Geometry: final body of the model. Coordinates: model frame, mm. A direction names the side the tool comes from. Give positions to 0.01 mm unless a question says otherwise; leave off trailing zeros. Loops run counter-clockwise (first coordinate to the right, second up) from the corner with the lowest first, then second, coordinate; pieces in that order, holes last. Notation, with made-up numbers: (26, -7.75) -> (74, -7.75) arc R14 cw to (74, 5.25) -> close; hole circle Ø5 at (-14.5, 3.25). An arc over 180 degrees is marked (long way). One line per question, with ' | ' between items. Start each with the question number.
Item 1: Set-up query: faces 1 (the cylindrical face through (10.24, -21.994, -4.224)), 2 (the flat face through (14, 22.2, 0)), 3 (the flat face through (-20.32, 0, -5)). Return all of +Z, -Z, +X, -X, +Y, -Y with unobstructed straight access to the full face (end or side cutting, diameter ignored); none if empty.
Item 2: Section D-D on y = 0. Return loops of the section in (x, z), then the cut area to 3 significant figures.
Item 3: Section B-B on x = -12. Give the number of separate pieces and of enclosed holes in the cut face, then the cut area to 3 significant figures.
Item 4: Section A-A on z = 24. Return loops of the section in (x, y).
Item 5: Material intervals for line 1 along X through (y, z) = (20, -3); line 2 along Y through (x, z) = (0, 18); line 3 along Z through (x, y) = (16.5, -7.5), sorted ascending. Write a range as [from, to].
Item 6: Section C-C on x = 0. Return loops of the section in (y, z) (3 decimals), then the cut area to 3 significant figures.
Item 7: Pin query (flat end, axial travel): P1, Ø7, axis at x = 12.065, y = 20.32, coming from the +Z side; P2, Ø10, axis at x = 13, y = -20, coming from the +Z side; P3, Ø3, axis at x = 12.065, y = 20.32, coming from the +Z side; P4, Ø1, axis at x = 5, y = 31, coming from the -Z side. Return the tip coordinate at first contact, or that it passes through.
Item 8: Mould query, pull axis Y, two halves, no side actions, for faces 4 (the flat face through (-10, 22, 0)), 5 (the flat face through (-1, -27, -2.54)), 6 (the cylindrical face through (35.09, 34.86, 26.46)). Classes: released by +Y, released by -Y, zero draft, split by the parting line, or undercut.
Autodesk Fusion 360 part; units mm, degrees
sketch "Sketch1" plane through (0, 0, 0) normal (0, 0, 1) x (1, 0, 0)
  line L0 (39.37, 39.37) -> (-39.37, 39.37)
  line L1 (-39.37, 39.37) -> (-39.37, -39.37)
  line L2 (-39.37, -39.37) -> (39.37, -39.37)
  line L3 (39.37, -39.37) -> (39.37, 39.37)
  line L4 (39.37, 39.37) -> (-39.37, -39.37) construction
  line L5 (-39.37, 39.37) -> (39.37, -39.37) construction
  dimension "d9" = 78.74
  dimension "d10" = 78.74
extrude "Extrude1" add sketch "Sketch1" along normal blind 50.8
sketch "Sketch2" plane through (0, 0, 50.8) normal (0, 0, 1) x (-1, 0, 0)
  line L0 (-39.37, 39.37) -> (-39.37, -39.37)
  line L1 (-39.37, -39.37) -> (39.37, -39.37)
  line L2 (39.37, -39.37) -> (39.37, 39.37)
  line L3 (39.37, 39.37) -> (-39.37, 39.37)
  circle A0 centre (0, 0) radius 36.83
  dimension "d13" = 73.66
extrude "Extrude2" cut sketch "Sketch2" against normal up to surface (50.8 mm away) contours A0
sketch "Sketch3" plane through (0, 0, 0) normal (0, 0, -1) x (1, 0, 0)
  circle A0 centre (0, 0) radius 36.83
  line L0 (39.37, -39.37) -> (39.37, 39.37)
  line L1 (39.37, 39.37) -> (-39.37, 39.37)
  line L2 (-39.37, 39.37) -> (-39.37, -39.37)
  line L3 (-39.37, -39.37) -> (39.37, -39.37)
  line L4 (-39.37, 39.37) -> (39.37, 39.37)
  line L5 (39.37, 39.37) -> (39.37, -39.37)
  line L6 (39.37, -39.37) -> (-39.37, -39.37)
  line L7 (-39.37, -39.37) -> (-39.37, 39.37)
extrude "Extrude3" add sketch "Sketch3" along normal blind 2.54 contours A0 | L0 L1 L2 L3 L4 L5 L6 L7
sketch "Sketch4" plane through (0, 0, -2.54) normal (0, 0, -1) x (1, 0, 0)
  line L0 (-39.37, -39.37) -> (39.37, -39.37)
  line L1 (39.37, -39.37) -> (39.37, 39.37)
  line L2 (39.37, 39.37) -> (-39.37, 39.37)
  line L3 (-39.37, 39.37) -> (-39.37, -39.37)
  line L4 (-20.32, 26.035) -> (20.32, 26.035)
  line L5 (20.32, 26.035) -> (20.32, -26.035)
  line L6 (20.32, -26.035) -> (-20.32, -26.035)
  line L7 (-20.32, -26.035) -> (-20.32, 26.035)
  line L8 (-20.32, 26.035) -> (20.32, -26.035) construction
  line L9 (20.32, 26.035) -> (-20.32, -26.035) construction
  dimension "d18" = 40.64
  dimension "d19" = 52.07
extrude "Extrude4" add sketch "Sketch4" along normal blind 5.7912 contours L4 L5 L6 L7
sketch "Sketch5" plane through (0, 0, -8.3312) normal (0, 0, -1) x (1, 0, 0)
  line L0 (-20.32, -26.035) -> (20.32, -26.035)
  line L1 (20.32, -26.035) -> (20.32, 26.035)
  line L2 (20.32, 26.035) -> (-20.32, 26.035)
  line L3 (-20.32, 26.035) -> (-20.32, -26.035)
  line L4 (-12.065, 20.32) -> (12.065, 20.32)
  line L5 (12.065, 20.32) -> (12.065, -20.32)
  line L6 (12.065, -20.32) -> (-12.065, -20.32)
  line L7 (-12.065, -20.32) -> (-12.065, 20.32)
  line L8 (-12.065, 20.32) -> (12.065, -20.32) construction
  line L9 (12.065, 20.32) -> (-12.065, -20.32) construction
  circle A0 centre (12.065, -20.32) radius 2.4765
  circle A1 centre (-12.065, -20.32) radius 2.4765
  circle A2 centre (-12.065, 20.32) radius 2.4765
  circle A3 centre (12.065, 20.32) radius 2.4765
  dimension "d23" = 24.13
  dimension "d24" = 40.64
  dimension "d26" = 4.953
  dimension "d27" = 4.953
  dimension "d28" = 4.953
  dimension "d29" = 4.953
extrude "Extrude5" cut sketch "Sketch5" against normal up to surface (59.1312 mm away) contours L4 L7 A2 | L4 L7 A2 | L4 L5 A3 | L4 L5 A3 | L6 L7 A1 | L6 L7 A1 | L5 L6 A0 | L5 L6 A0
sketch "Sketch6" plane through (0, 0, 0) normal (0, 0, 1) x (-1, 0, 0)
  circle A0 centre (12.065, -20.32) radius 2.4765
  circle A1 centre (12.065, 20.32) radius 2.4765
  circle A2 centre (-12.065, -20.32) radius 2.4765
  circle A3 centre (-12.065, 20.32) radius 2.4765
  circle A4 centre (0, 0) radius 36.83
  line L0 (-12.065, 20.32) -> (12.065, 20.32)
  line L1 (12.065, 20.32) -> (12.065, -20.32)
  line L2 (12.065, -20.32) -> (-12.065, -20.32)
  line L3 (-12.065, -20.32) -> (-12.065, 20.32)
  circle A5 centre (-12.065, 20.32) radius 4.445
  circle A6 centre (12.065, 20.32) radius 4.445
  circle A7 centre (-12.065, -20.32) radius 4.445
  circle A8 centre (12.065, -20.32) radius 4.445
  dimension "d33" = 8.89
  dimension "d34" = 8.89
  dimension "d35" = 8.89
  dimension "d36" = 8.89
extrude "Extrude6" add sketch "Sketch6" along normal blind 6.35 contours L0 L1 L2 L3 A5 A6 A7 A8 | A4
extrude "Extrude7" add 1 faces at (29.7771, -31.0719, 50.8) along direction (0, 0, 1) blind 6.35
fillet "Fillet1" radius 15 4 edges at (39.37, -39.37, 27.305) (39.37, 39.37, 27.305) (-39.37, -39.37, 27.305) (-39.37, 39.37, 27.305)
fillet "Fillet2" radius 2.5 8 edges at (-34.9766, 34.9766, 57.15) (-39.37, 0, 57.15) (-34.9766, -34.9766, 57.15) (0, -39.37, 57.15) (34.9766, -34.9766, 57.15) (39.37, 0, 57.15) (34.9766, 34.9766, 57.15) (0, 39.37, 57.15)
equation "CupBaseDiameter = 2.7 in"
equation "CupHeight = 2 in"
equation "CupTopDiameter = 2.9 in"
equation "HoleDistanceLength = 0.95 in"
equation "HoleDistanceWidth = 1.6 in"
equation "BaseLength = 1.6 in"
equation "BaseWidth = 2.05 in"
equation "CupTop = CupTopDiameter + 0.2 in"
equation "d9 = CupTop"
equation "d10 = CupTop"
equation "d11 = CupHeight"
equation "d13 = CupTopDiameter"
equation "d18 = BaseLength"
equation "d19 = BaseWidth"
equation "BaseHeight = 0.228 in"
equation "d21 = BaseHeight"
equation "d23 = HoleDistanceLength"
equation "d24 = HoleDistanceWidth"
equation "ScrewHoleDiameter = 0.195 in"
equation "d26 = ScrewHoleDiameter"
equation "d27 = ScrewHoleDiameter"
equation "d28 = ScrewHoleDiameter"
equation "d29 = ScrewHoleDiameter"
equation "ScrewTopDiamater = 0.35 in"
equation "d33 = ScrewTopDiamater"
equation "d34 = ScrewTopDiamater"
equation "d35 = ScrewTopDiamater"
equation "d36 = ScrewTopDiamater"
Result sheet:
1) face 1: +Z, -Z | face 2: +Z | face 3: -Z, -X, +Y, -Y
2) outline: (-39.37, -2.54) -> (-20.32, -2.54) -> (-20.32, -8.33) -> (20.32, -8.33) -> (20.32, -2.54) -> (39.37, -2.54) -> (39.37, 54.65) arc R2.5 ccw to (36.87, 57.15) -> (36.83, 57.15) -> (36.83, 6.35) -> (-36.83, 6.35) -> (-36.83, 57.15) -> (-36.87, 57.15) arc R2.5 ccw to (-39.37, 54.65) -> close | area: 1,190 mm²
3) separate pieces: 3 | enclosed holes: 0 | area: 1,270 mm²
4) outline: (-39.37, -24.37) arc R15 ccw to (-24.37, -39.37) -> (24.37, -39.37) arc R15 ccw to (39.37, -24.37) -> (39.37, 24.37) arc R15 ccw to (24.37, 39.37) -> (-24.37, 39.37) arc R15 ccw to (-39.37, 24.37) -> close; hole circle Ø73.66 at (0, 0)
5) line 1: x = [-20.32, -14.52], [-9.61, 9.61], [14.52, 20.32] | line 2: y = [-39.37, -36.83], [36.83, 39.37] | line 3: z = [-8.33, 6.35]
6) outline: (-39.37, -2.54) -> (-26.035, -2.54) -> (-26.035, -8.331) -> (26.035, -8.331) -> (26.035, -2.54) -> (39.37, -2.54) -> (39.37, 54.65) arc R2.5 ccw to (36.87, 57.15) -> (36.83, 57.15) -> (36.83, 6.35) -> (-36.83, 6.35) -> (-36.83, 57.15) -> (-36.87, 57.15) arc R2.5 ccw to (-39.37, 54.65) -> close | area: 1,260 mm²
7) P1: stops at z = 0 | P2: stops at z = 6.35 | P3: passes through | P4: stops at z = -2.54
8) face 4: undercut | face 5: zero draft | face 6: released by +Y
